Design review of the part built by this model. Coordinates are the model's own, in mm. A direction names the side the tool comes from. Coordinates: 2 decimals unless noted, no trailing zeros. Write each loop counter-clockwise with the first axis right and the second up, starting at its lowest first coordinate (ties: lowest second). Pieces come first, ordered by that corner, then holes. Notation, with made-up numbers: (88, 0) -> (130, 0) arc R5 cw to (130, 7) -> close; hole circle Ø9 at (49, 75). An arc over 180 degrees is marked (long way). Answer in a Markdown table with one row per item. Add a question column.
Item 1: For faces 4 (the face through (-6, 22, -24.3)), 5 (the face through (-4, -12, -24.3)), 6 (the face through (1, 20, 21.3)), 7 (the face through (-6, 24.3, 0)), 8 (the face through (-6, 21.3, 0)), list the 3-axis set-ups (+Z, -Z, +X, -X, +Y, -Y) from which the entire face can be reached by the end or side of a thin tool; tool diameter is ignored.
Item 2: Take a section at B-B, the plane z = -32.5. Write out the cut boundary in (x, y), and give its area (3 significant figures).
Item 3: Clearance check with flat-ended pins moving along their axes: P1, Ø4, axis at x = -3, z = 4, coming from the -Y side; P2, Ø1.9, axis at y = 5, z = 26, coming from the +X side; P3, Ø9, axis at y = 32, z = 8, coming from the -X side; P4, Ø9.5, axis at x = -8.5, z = 5, coming from the +Y side. State where each tip first meets the part, or that it passes through.
Item 4: Draft analysis for pull direction Y (two halves, no side actions). For faces 1 (the face through (-6, 0, -21.3)), 2 (the face through (1.97, -16.68, 14.42)), 3 (the face through (1, -21.3, -5)), state which applies: released by +Y, released by -Y, zero draft, split by the parting line, or undercut.
Item 5: Take a section at A-A, the plane y = 15.5. Write out the cut boundary in (x, z).
Item 6: Take a section at D-D, the plane y = -2. Write out the cut boundary in (x, z).
Item 7: To check wall thickness, follow line 1 (Z direction, x = 1.1, y = 0); line 2 (Y direction, x = -7.5, z = -11); line 3 (Z direction, x = -2, y = -10). State the ranges of each line that lie inside material, in increasing order.
Item 8: Take a section at C-C, the plane x = -10.5. Write out the cut boundary in (y, z).
Autodesk Fusion 360 part; units mm, degrees
sketch "motor_mount" plane through (0, 0, 0) normal (1, 0, 0) x (0, 1, 0)
  circle A0 centre (0, 0) radius 11.25
  line L0 (15.5, 15.5) -> (-15.5, 15.5) construction
  line L1 (-15.5, 15.5) -> (-15.5, -15.5) construction
  line L2 (-15.5, -15.5) -> (15.5, -15.5) construction
  line L3 (15.5, -15.5) -> (15.5, 15.5) construction
  line L4 (15.5, 15.5) -> (-15.5, -15.5) construction
  line L5 (-15.5, 15.5) -> (15.5, -15.5) construction
  line L6 (21.3, 21.3) -> (-21.3, 21.3)
  line L7 (-21.3, 21.3) -> (-21.3, -21.3)
  line L8 (-21.3, -21.3) -> (21.3, -21.3)
  line L9 (21.3, -21.3) -> (21.3, 21.3)
  line L10 (21.3, 21.3) -> (-21.3, -21.3) construction
  line L11 (-21.3, 21.3) -> (21.3, -21.3) construction
  line L12 (-21.3, -21.3) -> (21.3, -21.3)
  line L13 (-21.3, -21.3) -> (21.3, -21.3)
  line L14 (21.3, -24.3) -> (-21.3, -24.3)
  line L15 (-21.3, -24.3) -> (-21.3, -21.3)
  circle A1 centre (-15.5, 15.5) radius 1.6
  circle A2 centre (15.5, 15.5) radius 1.6
  circle A3 centre (-15.5, -15.5) radius 1.6
  circle A4 centre (15.5, -15.5) radius 1.6
  circle A5 centre (36.8, -32.5) radius 1.6
  circle A6 centre (5.8, -32.5) radius 1.6
  line L16 (5.8, -32.5) -> (36.8, -32.5) construction
  line L17 (0, -24.3) -> (-3, -24.3)
  line L18 (-3, -24.3) -> (-3, -43.3)
  line L19 (-3, -43.3) -> (0, -43.3)
  line L20 (0, -43.3) -> (0, -24.3)
  line L21 (0, -43.3) -> (42.6, -43.3)
  line L22 (42.6, -43.3) -> (42.6, -24.3)
  line L23 (42.6, -24.3) -> (21.3, -24.3)
  line L24 (21.3, -21.3) -> (42.6, -21.3)
  line L25 (42.6, -21.3) -> (42.6, -24.3)
  line L26 (21.3, 21.3) -> (24.3, 21.3)
  line L27 (24.3, 21.3) -> (24.3, -21.3)
  line L28 (24.3, -21.3) -> (21.3, -21.3)
  line L29 (21.3, -21.3) -> (21.3, 21.3)
  line L30 (24.3, 21.3) -> (42.6, -21.3)
  line L31 (0, 21.3) -> (-8, 21.3)
  line L32 (-8, 21.3) -> (8, 21.3)
  line L33 (8, 21.3) -> (8, 29.9)
  line L34 (8, 29.9) -> (-8, 29.9)
  line L35 (-8, 29.9) -> (-8, 21.3)
  circle A7 centre (-5, 26) radius 1.6
  circle A8 centre (5, 26) radius 1.6
  dimension "d1" = 22.5
  dimension "d2" = 31
  dimension "d3" = 31
  dimension "d5" = 42.6
  dimension "d6" = 42.6
  dimension "d8" = 3
  dimension "d9" = 3.2
  dimension "d10" = 3.2
  dimension "d11" = 3.2
  dimension "d12" = 3.2
  dimension "d13" = 3.2
  dimension "d14" = 3.2
  dimension "d267" = 31
  dimension "d268" = 3
  dimension "d269" = 19
  dimension "d270" = 42.6
  dimension "d271" = 3
  dimension "d286" = 8
  dimension "d287" = 16
  dimension "d288" = 8.6
  dimension "d323" = 3.2
  dimension "d324" = 3.2
extrude "Extrude1" add sketch "motor_mount" along normal blind 4 makes body 1
extrude "Extrude2" add sketch "motor_mount" against normal blind 12 contours L9 L24 L26 L27 L28 L29 | L8 L12 L13 L14 L15 L17 L23 L24 L25 L28 | L14 L17 L18 L19 L20 bodies 1
mirror "Mirror1" about plane through (0, 0, 0) normal (0, 1, 0) of bodies 1 makes body 2
hidden bodies 2
equation "pen_min_diam = 8 mm"
equation "pen_max_diam = 13 mm"
equation "pen_holder_diam = 17 mm"
equation "pen_shaft_diam = 23 mm"
equation "pen_sled_diam = 50 mm"
equation "pen_bearing_tolerance = 0.7 mm"
equation "pen_support_diam = 36 mm"
equation "pen_shaft_tolerance = 0.8 mm"
equation "sled_thickness = 4 mm"
equation "bearing_offset_ring_thickness = 0.5 mm"
equation "assembly_tolerance = 0.2 mm"
equation "bearing_1_plane = sled_thickness + bearing_offset_ring_thickness + assembly_tolerance"
equation "bearing_thickness = 3.6 mm"
equation "bearing_2_plane = bearing_1_plane + bearing_thickness + assembly_tolerance"
equation "bearing_cap_threaded_thickness = 4 mm"
equation "bearing_cap_supported_thickness = 4 mm"
equation "bearing_cap_height = 20 mm"
Answers:
| question | item | result |
|---|---|---|
| 1 | face 4 | -Z, -X, +Y |
| 1 | face 5 | -Z, +X, -X, -Y |
| 1 | face 6 | +Z, +X, -X, +Y |
| 1 | face 7 | +Z, -X, +Y |
| 1 | face 8 | +Z, -X, -Y |
| 2 | outline | (-12, -3) -> (4, -3) -> (4, 4.2) -> (0, 4.2) -> (0, 0) -> (-12, 0) -> close; (0, 7.4) -> (4, 7.4) -> (4, 35.2) -> (0, 35.2) -> close; (0, 38.4) -> (4, 38.4) -> (4, 42.6) -> (0, 42.6) -> close |
| 2 | area | 193 mm^2 |
| 3 | P1 | stops at y = 21.3 |
| 3 | P2 | passes through |
| 3 | P3 | stops at x = 0 |
| 3 | P4 | stops at y = 24.3 |
| 4 | face 1 | zero draft |
| 4 | face 2 | undercut |
| 4 | face 3 | released by -Y |
| 5 | outline | (-12, -24.3) -> (0, -24.3) -> (0, -43.3) -> (4, -43.3) -> (4, -17.1) -> (0, -17.1) -> (0, -21.3) -> (-12, -21.3) -> close; (0, -13.9) -> (4, -13.9) -> (4, 13.9) -> (0, 13.9) -> close; (0, 17.1) -> (4, 17.1) -> (4, 21.3) -> (0, 21.3) -> close |
| 6 | outline | (-12, -43.3) -> (4, -43.3) -> (4, -11.07) -> (0, -11.07) -> (0, -21.3) -> (-12, -21.3) -> close; (0, 11.07) -> (4, 11.07) -> (4, 29.9) -> (0, 29.9) -> close |
| 7 | line 1 | z = -43.3 to -11.25, 11.25 to 29.9 |
| 7 | line 2 | y = 21.3 to 24.3 |
| 7 | line 3 | z = -24.3 to -21.3 |
| 8 | outline | (-21.3, -24.3) -> (-3, -24.3) -> (-3, -43.3) -> (0, -43.3) -> (0, -24.3) -> (42.6, -24.3) -> (42.6, -21.3) -> (24.3, -21.3) -> (24.3, 21.3) -> (21.3, 21.3) -> (21.3, -21.3) -> (-21.3, -21.3) -> close |
